Source: CAD feature listing. Evaluate the final solid. Frame: model axes, mm. Face numbers are marked on the shaded views. A direction names the side the tool comes from. Give positions to 0.01 mm unless a question says otherwise; leave off trailing zeros. Order: outer loops, then holes, each group sorted by start corner. A loop starts at its lowest first (then second) coordinate and runs counter-clockwise, first axis right, second up. Notation, with made-up numbers: (-22.75, -19) - (9.25, -19) arc R10 ccw to (9.25, -10) - close; hole circle Ø6 at (19.25, -16.75). An arc over 180 degrees is marked (long way). Write each question's results on one line, items separated by ' | '. Start each with the question number.
Item 1: Mould query, pull axis X, two halves, no side actions, for the marked faces 1, 2 and 3. Classes: released by +X, released by -X, zero draft, split by the parting line, or undercut.
Item 2: Set-up query: the marked faces 4, 5, 6 and 7. Return all of +Z, -Z, +X, -X, +Y, -Y with unobstructed straight access to the full face (end or side cutting, diameter ignored); none if empty.
Item 3: Section D-D on x = -7.25. Output: boundary loops of the cut face in (y, z), and give its area (3 significant figures).
Item 4: Section A-A on y = 21. Output: boundary loops of the cut face in (x, z).
Item 5: Contact query for flat-ended pins moving along their axis: pin 1 Ø2.5 at (y, z) = (-29.99, 2) entering from +X; pin 2 Ø1.3 at (y, z) = (-15, 3.5) entering from -X; pin 3 Ø2.5 at (y, z) = (30.5, 2.5) entering from +X. Output: stop coordinate, or through.
Item 6: Section C-C on y = -12. Output: boundary loops of the cut face in (x, z).
Item 7: Section B-B on x = -1.25. Output: boundary loops of the cut face in (y, z).
Item 8: Line query: line 1 along Y through (x, z) = (-1, 2); line 2 along X through (y, z) = (9.5, 1.2); line 3 along X through (y, z) = (26, 4.2). Output: solid intervals per line, ascending.
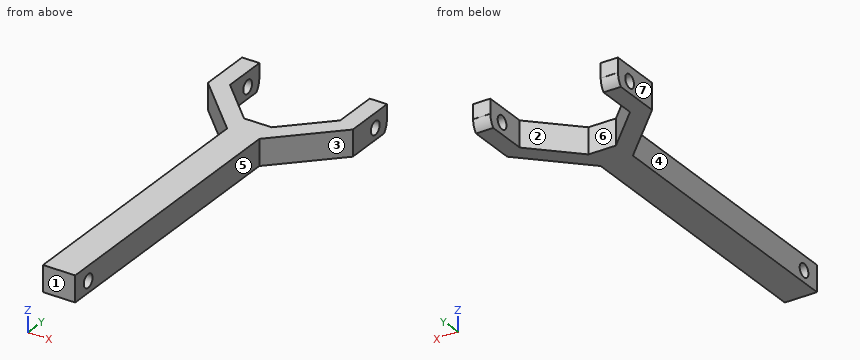
```python
from build123d import *

# Parameters (mm, degrees)
EXTRUDE_1_DEPTH          = 4.5
CUT_EXTRUDE_1_DEPTH      = 100
CUT_EXTRUDE_1_DEPTH_BACK = 100
SKETCH_2_R               = 1.150000595
SKETCH_2_R_2             = 1.150000006
CUT_EXTRUDE_2_DEPTH      = 100
CUT_EXTRUDE_2_DEPTH_BACK = 10


with BuildPart() as part:
    # 草图1 → 凸台-拉伸1 (new body)
    with BuildSketch(Plane.XY):
        Polygon((-3.663147943, -33.4008975), (1.914578421, -33.4008975), (1.914578421, 14.960326674), (11.675714921, 24.721462524), (11.675714921, 33.692325595), (8.675714, 33.692325595), (8.675714, 25.964104178), (1.514824851, 18.803215506), (-3.263396279, 18.803215506), (-10.424284951, 25.964104655), (-10.424284951, 33.692326072), (-13.424284951, 33.692326072), (-13.424284951, 24.721463921), (-3.663147943, 14.960326674), align=None)
    extrude(amount=EXTRUDE_1_DEPTH)

    # 草图2 → 切除-拉伸1 (cut, two sides: drawn at the far end of the back side and taken through both)
    with BuildSketch(Plane(origin=(0, 0, 0), x_dir=(0, 0, -1), z_dir=(1, 0, 0)).offset(-CUT_EXTRUDE_1_DEPTH_BACK)):
        with Locations(Location((-2.000000723, -29.993528863, 0), (0, 0, 180))):
            Circle(SKETCH_2_R)
        with Locations(Location((-2.000000233, 30.610505435, 0), (0, 0, 180))):
            Circle(SKETCH_2_R_2)
    extrude(amount=CUT_EXTRUDE_1_DEPTH + CUT_EXTRUDE_1_DEPTH_BACK, mode=Mode.SUBTRACT)

    # 草图3 → 切除-拉伸2 (cut, two sides: drawn at the far end of the back side and taken through both)
    with BuildSketch(Plane(origin=(-10.424284951, 0, 0), x_dir=(0, 0, -1), z_dir=(1, 0, 0)).offset(-CUT_EXTRUDE_2_DEPTH_BACK)):
        with BuildLine():
            Line((-2.000000233, 33.665271008), (-2.000000233, 37.690968831))
            ThreePointArc((-2.000000233, 37.690968831), (3.006643449, 35.617149116), (5.080463163, 30.610505435))
            Line((5.080463163, 30.610505435), (1.05476534, 30.610505435))
            ThreePointArc((1.05476534, 30.610505435), (0.160045219, 32.770550887), (-2.000000233, 33.665271008))
        make_face()
    extrude(amount=CUT_EXTRUDE_2_DEPTH + CUT_EXTRUDE_2_DEPTH_BACK, mode=Mode.SUBTRACT)


solid = part.part
```
Evaluation:
1) face 1: zero draft | face 2: undercut | face 3: released by +X
2) face 4: +Z, -Z, -X, -Y | face 5: +Z, -Z, +X, -Y | face 6: +Z, -Z, +Y | face 7: +Z, -Z, -X, +Y, -Y
3) outline: (18.55, 0) - (22.79, 0) - (22.79, 4.5) - (18.55, 4.5) - close | area: 19.1 mm^2
4) outline: (-9.7, 0) - (-5.46, 0) - (-5.46, 4.5) - (-9.7, 4.5) - close; (3.71, 0) - (7.95, 0) - (7.95, 4.5) - (3.71, 4.5) - close
5) pin 1: stops at x = 1.91 | pin 2: stops at x = -3.66 | pin 3: stops at x = 11.68
6) outline: (-3.66, 0) - (1.91, 0) - (1.91, 4.5) - (-3.66, 4.5) - close
7) outline: (-33.4, 0) - (18.8, 0) - (18.8, 4.5) - (-33.4, 4.5) - close; hole circle Ø2.3 at (-29.99, 2)
8) line 1: y = -33.4 to -31.14, -28.84 to 18.8 | line 2: x = -3.66 to 1.91 | line 3: x = -13.42 to -10.42, 8.68 to 11.68
